from build123d import *

# Parameters (mm, degrees)
SKETCH1_W           = 80
SKETCH1_H           = 150
SKETCH1_W_2         = 66
SKETCH1_H_2         = 136
BOSS_EXTRUDE1_DEPTH = 7
SKETCH2_W           = 66
SKETCH2_H           = 36
BOSS_EXTRUDE2_DEPTH = 7
SKETCH3_R           = 5.5
CUT_EXTRUDE1_DEPTH  = 86.287748241
SKETCH4_R           = 6.05
CUT_EXTRUDE2_DEPTH  = 5.6
SKETCH5_R           = 11
CUT_EXTRUDE3_DEPTH  = 3
SKETCH6_R           = 1.6
CUT_EXTRUDE4_DEPTH  = 86.287748241
SKETCH7_W           = 50
SKETCH7_H           = 38
CUT_EXTRUDE5_DEPTH  = 1
SKETCH8_R           = 3
CUT_EXTRUDE6_DEPTH  = 3
SKETCH9_R           = 1.35
CUT_EXTRUDE7_DEPTH  = 86.287748241
SKETCH10_R          = 2.4
CUT_EXTRUDE8_DEPTH  = 5
CHAMFER1_SIZE       = 2
SKETCH11_W          = 66
SKETCH11_H          = 30.5
BOSS_EXTRUDE3_DEPTH = 7
SKETCH12_R          = 1.35
CUT_EXTRUDE9_DEPTH  = 86.287748241
SKETCH13_R          = 2.4
CUT_EXTRUDE10_DEPTH = 5


with BuildPart() as part:
    # Sketch1 → Boss-Extrude1 (new body)
    with BuildSketch(Plane.XY):
        Rectangle(SKETCH1_W, SKETCH1_H)
        Rectangle(SKETCH1_W_2, SKETCH1_H_2, mode=Mode.SUBTRACT)
    extrude(amount=BOSS_EXTRUDE1_DEPTH)

    # Sketch2 → Boss-Extrude2 (add)
    with BuildSketch(Plane.XY.offset(7)):
        with Locations((0, -50)):
            Rectangle(SKETCH2_W, SKETCH2_H)
    extrude(amount=-BOSS_EXTRUDE2_DEPTH)

    # Sketch3 → Cut-Extrude1 (cut, through all)
    with BuildSketch(Plane(origin=(0, 0, 0), x_dir=(-1, 0, 0), z_dir=(0, 0, -1))):
        with Locations((0, -55)):
            Circle(SKETCH3_R)
    extrude(amount=-CUT_EXTRUDE1_DEPTH, mode=Mode.SUBTRACT)

    # Sketch4 → Cut-Extrude2 (cut)
    with BuildSketch(Plane(origin=(0, 0, 0), x_dir=(-1, 0, 0), z_dir=(0, 0, -1))):
        with Locations((0, -55)):
            Circle(SKETCH4_R)
    extrude(amount=-CUT_EXTRUDE2_DEPTH, mode=Mode.SUBTRACT)

    # Sketch5 → Cut-Extrude3 (cut)
    with BuildSketch(Plane(origin=(0, 0, 0), x_dir=(-1, 0, 0), z_dir=(0, 0, -1))):
        with Locations((0, -55)):
            Circle(SKETCH5_R)
    extrude(amount=-CUT_EXTRUDE3_DEPTH, mode=Mode.SUBTRACT)

    # Sketch6 → Cut-Extrude4 (cut, through all)
    with BuildSketch(Plane(origin=(0, 0, 0), x_dir=(-1, 0, 0), z_dir=(0, 0, -1))):
        with Locations((-13, -42)):
            Circle(SKETCH6_R)
        with Locations((13, -42)):
            Circle(SKETCH6_R)
        with Locations((13, -68)):
            Circle(SKETCH6_R)
        with Locations((-13, -68)):
            Circle(SKETCH6_R)
    extrude(amount=-CUT_EXTRUDE4_DEPTH, mode=Mode.SUBTRACT)

    # Sketch7 → Cut-Extrude5 (cut)
    with BuildSketch(Plane(origin=(0, 0, 0), x_dir=(-1, 0, 0), z_dir=(0, 0, -1))):
        with Locations((0, -55)):
            Rectangle(SKETCH7_W, SKETCH7_H)
    extrude(amount=-CUT_EXTRUDE5_DEPTH, mode=Mode.SUBTRACT)

    # Sketch8 → Cut-Extrude6 (cut)
    with BuildSketch(Plane.XY.offset(7)):
        with Locations((-13, -42)):
            Circle(SKETCH8_R)
        with Locations((13, -42)):
            Circle(SKETCH8_R)
        with Locations((13, -68)):
            Circle(SKETCH8_R)
        with Locations((-13, -68)):
            Circle(SKETCH8_R)
    extrude(amount=-CUT_EXTRUDE6_DEPTH, mode=Mode.SUBTRACT)

    # Sketch9 → Cut-Extrude7 (cut, through all)
    with BuildSketch(Plane.XY.offset(7)):
        with Locations((-36.5, 71.5)):
            Circle(SKETCH9_R)
        with Locations((36.5, 71.5)):
            Circle(SKETCH9_R)
        with Locations((-36.5, -71.5)):
            Circle(SKETCH9_R)
        with Locations((36.5, -71.5)):
            Circle(SKETCH9_R)
        with Locations((-36.5, 35.5)):
            Circle(SKETCH9_R)
        with Locations((36.5, 35.5)):
            Circle(SKETCH9_R)
        with Locations((36.5, -26.5)):
            Circle(SKETCH9_R)
        with Locations((-36.5, -26.5)):
            Circle(SKETCH9_R)
    extrude(amount=-CUT_EXTRUDE7_DEPTH, mode=Mode.SUBTRACT)

    # Sketch10 → Cut-Extrude8 (cut)
    with BuildSketch(Plane.XY.offset(7)):
        with Locations((-36.5, 71.5)):
            Circle(SKETCH10_R)
        with Locations((36.5, 35.5)):
            Circle(SKETCH10_R)
        with Locations((-36.5, 35.5)):
            Circle(SKETCH10_R)
        with Locations((36.5, 71.5)):
            Circle(SKETCH10_R)
        with Locations((-36.5, -71.5)):
            Circle(SKETCH10_R)
        with Locations((36.5, -71.5)):
            Circle(SKETCH10_R)
        with Locations((-36.5, -26.5)):
            Circle(SKETCH10_R)
        with Locations((36.5, -26.5)):
            Circle(SKETCH10_R)
    extrude(amount=-CUT_EXTRUDE8_DEPTH, mode=Mode.SUBTRACT)

    # Chamfer1
    # the kernel refuses this chamfer: 2 mm, written as the material it takes off along each edge
    with BuildSketch(Plane(origin=(-40, 80.143365976, 7), x_dir=(-0.027495876610585623, 0, -0.9996219169112968), z_dir=(0, -1, 0)), Plane(origin=(40, -80.143365976, 7), x_dir=(0.027495876610585623, 0, -0.9996219169112968), z_dir=(0, 1, 0))) as chamfer1_piece_1:
        Polygon((CHAMFER1_SIZE * 0.999621916911, CHAMFER1_SIZE * 0.0274958766106), (-CHAMFER1_SIZE * 0.0274958766106, CHAMFER1_SIZE * 0.999621916911), (0, 0), align=None)
    extrude(amount=160.286731952, mode=Mode.SUBTRACT)

    # Sketch11 → Boss-Extrude3 (add)
    with BuildSketch(Plane.XY.offset(7)):
        with Locations((0, -16.75)):
            Rectangle(SKETCH11_W, SKETCH11_H)
    extrude(amount=-BOSS_EXTRUDE3_DEPTH)

    # Sketch12 → Cut-Extrude9 (cut, through all)
    with BuildSketch(Plane.XY.offset(7)):
        with Locations((-20, 71.5)):
            Circle(SKETCH12_R)
        with Locations((20, 71.5)):
            Circle(SKETCH12_R)
    extrude(amount=-CUT_EXTRUDE9_DEPTH, mode=Mode.SUBTRACT)

    # Sketch13 → Cut-Extrude10 (cut)
    with BuildSketch(Plane.XY.offset(7)):
        with Locations((-20, 71.5)):
            Circle(SKETCH13_R)
        with Locations((20, 71.5)):
            Circle(SKETCH13_R)
    extrude(amount=-CUT_EXTRUDE10_DEPTH, mode=Mode.SUBTRACT)


solid = part.part
Part model, mm, in its own coordinate system. A direction names the side the tool comes from. Give positions to 0.01 mm unless a question says otherwise; leave off trailing zeros. Loops run counter-clockwise (first coordinate to the right, second up) from the corner with the lowest first, then second, coordinate; pieces in that order, holes last. Notation, with made-up numbers: (18, -1.75) -> (31, -1.75) arc R7 ccw to (31, 11.25) -> close; hole circle Ø8 at (-24.5, 73.25). An arc over 180 degrees is marked (long way). Write each question's results on one line, items separated by ' | '. Start each with the question number.
Q1. Band-saw the part on B-B on y = 48. List the corners of the cut face in (x, z).
Q2. Pin check, flat tips, straight feed: P1, Ø4, axis at x = -13, y = -68, coming from the +Z side; P2, Ø4, axis at x = -36.5, y = -71.5, coming from the +Z side; P3, Ø1, axis at y = -50, z = 6.5, coming from the -X side. Stop position of each tip, or through.
Q3. Band-saw the part on A-A on y = -42. List the corners of the cut face in (x, z).
Q4. Wall check: L1, parallel to Y at x = 36.5, z = 0.9; L2, parallel to X at y = -68, z = 2; L3, parallel to Y at x = 13, z = 3.45. Give the ranges that are in metal, low to high.
Q5. Which spindle directions (+Z, -Z, +X, -X, +Y, -Y) get a long thin tool onto all of the face, cutting with end or side? Do faces 4 (the face through (-34.21, 72.22, 4.54)), 5 (the face through (0, -1.5, 4)), 6 (the face through (-2.79, -60.37, 4.28)), 7 (the face through (-1, -75, 3)). Say none if no direction does.
Q6. Pull direction X, two halves, no side cores. Call faces 1 (the face through (38, -73, 2)), 2 (the face through (-1, 75, 3)), 3 (the face through (-40, -1, 2)): +X half, -X half, draft (parallel to the pull), parting line (faces both ways), or undercut.
Q7. Band-saw the part on C-C on x = 13. List the corners of the cut face in (y, z).
Results are:
1) outline: (-40, 0) -> (-33, 0) -> (-33, 7) -> (-38, 7) -> (-40, 5) -> close; (33, 0) -> (40, 0) -> (40, 5) -> (38, 7) -> (33, 7) -> close
2) P1: stops at z = 4 | P2: stops at z = 2 | P3: stops at x = -39
3) outline: (-40, 0) -> (-25, 0) -> (-25, 1) -> (-14.6, 1) -> (-14.6, 4) -> (-16, 4) -> (-16, 7) -> (-38, 7) -> (-40, 5) -> close; (-11.4, 1) -> (11.4, 1) -> (11.4, 4) -> (10, 4) -> (10, 7) -> (-10, 7) -> (-10, 4) -> (-11.4, 4) -> close; (14.6, 1) -> (25, 1) -> (25, 0) -> (40, 0) -> (40, 5) -> (38, 7) -> (16, 7) -> (16, 4) -> (14.6, 4) -> close
4) L1: y = -75 to -72.85, -70.15 to -27.85, -25.15 to 34.15, 36.85 to 70.15, 72.85 to 75 | L2: x = -40 to -14.6, -11.4 to 11.4, 14.6 to 40 | L3: y = -75 to -69.6, -66.4 to -43.6, -40.4 to -1.5, 68 to 75
5) face 4: +Z | face 5: +Z, -Z | face 6: -Z | face 7: +Z, -Z, +X, -X, -Y
6) face 1: undercut | face 2: draft | face 3: -X half
7) outline: (-75, 0) -> (-74, 0) -> (-74, 1) -> (-69.6, 1) -> (-69.6, 4) -> (-71, 4) -> (-71, 7) -> (-75, 7) -> close; (-66.4, 1) -> (-43.6, 1) -> (-43.6, 4) -> (-45, 4) -> (-45, 7) -> (-65, 7) -> (-65, 4) -> (-66.4, 4) -> close; (-40.4, 1) -> (-36, 1) -> (-36, 0) -> (-1.5, 0) -> (-1.5, 7) -> (-39, 7) -> (-39, 4) -> (-40.4, 4) -> close; (68, 0) -> (75, 0) -> (75, 7) -> (68, 7) -> close
